Read the model definition and answer for the solid it produces. Units are mm, in the model's axes. Coordinates: 2 decimals unless noted, no trailing zeros. Order: outer loops, then holes, each group sorted by start corner. A loop starts at its lowest first (then second) coordinate and runs counter-clockwise, first axis right, second up.
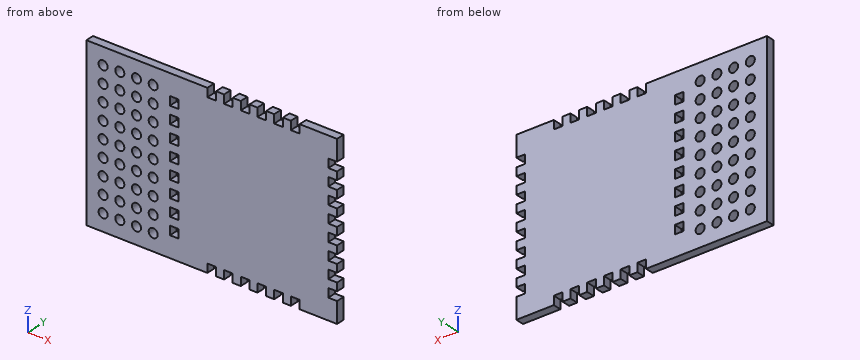
```python
from build123d import *

# Parameters (mm, degrees)
SKETCH1_W           = 127
SKETCH1_H           = 127
BOSS_EXTRUDE1_DEPTH = 6.35
SKETCH2_W           = 6.604
SKETCH2_H           = 6.477
SKETCH2_H_2         = 6.604
CUT_EXTRUDE1_DEPTH  = 91.02678768
SKETCH3_W           = 63.5
SKETCH3_H           = 127
SKETCH3_R           = 3.429
BOSS_EXTRUDE2_DEPTH = 6.35


with BuildPart() as part:
    # Sketch1 → Boss-Extrude1 (new body)
    with BuildSketch(Plane(origin=(0, 0, 0), x_dir=(1, 0, 0), z_dir=(0, 1, 0))):
        Rectangle(SKETCH1_W, SKETCH1_H)
    extrude(amount=BOSS_EXTRUDE1_DEPTH)

    # Sketch2 → Cut-Extrude1 (cut, through all)
    with BuildSketch(Plane(origin=(0, 6.35, 0), x_dir=(1, 0, 0), z_dir=(0, 1, 0))):
        with Locations((-31.75, -60.2615)):
            Rectangle(SKETCH2_W, SKETCH2_H)
        with Locations((-19.05, -60.2615)):
            Rectangle(SKETCH2_W, SKETCH2_H)
        with Locations((-6.35, -60.2615)):
            Rectangle(SKETCH2_W, SKETCH2_H)
        with Locations((6.35, -60.2615)):
            Rectangle(SKETCH2_W, SKETCH2_H)
        with Locations((19.05, -60.2615)):
            Rectangle(SKETCH2_W, SKETCH2_H)
        with Locations((31.75, -60.2615)):
            Rectangle(SKETCH2_W, SKETCH2_H)
        with Locations((31.75, 60.2615)):
            Rectangle(SKETCH2_W, SKETCH2_H)
        with Locations((19.05, 60.2615)):
            Rectangle(SKETCH2_W, SKETCH2_H)
        with Locations((6.35, 60.2615)):
            Rectangle(SKETCH2_W, SKETCH2_H)
        with Locations((-6.35, 60.2615)):
            Rectangle(SKETCH2_W, SKETCH2_H)
        with Locations((-19.05, 60.2615)):
            Rectangle(SKETCH2_W, SKETCH2_H)
        with Locations((-31.75, 60.2615)):
            Rectangle(SKETCH2_W, SKETCH2_H)
        with Locations((-60.198, 31.75)):
            Rectangle(SKETCH2_W, SKETCH2_H_2)
        with Locations((-60.198, 19.05)):
            Rectangle(SKETCH2_W, SKETCH2_H_2)
        with Locations((-60.198, 6.35)):
            Rectangle(SKETCH2_W, SKETCH2_H_2)
        with Locations((-60.198, -6.35)):
            Rectangle(SKETCH2_W, SKETCH2_H_2)
        with Locations((-60.198, -19.05)):
            Rectangle(SKETCH2_W, SKETCH2_H_2)
        with Locations((-60.198, -31.75)):
            Rectangle(SKETCH2_W, SKETCH2_H_2)
        with Locations((60.198, -31.75)):
            Rectangle(SKETCH2_W, SKETCH2_H_2)
        with Locations((60.198, -19.05)):
            Rectangle(SKETCH2_W, SKETCH2_H_2)
        with Locations((60.198, -6.35)):
            Rectangle(SKETCH2_W, SKETCH2_H_2)
        with Locations((60.198, 6.35)):
            Rectangle(SKETCH2_W, SKETCH2_H_2)
        with Locations((60.198, 19.05)):
            Rectangle(SKETCH2_W, SKETCH2_H_2)
        with Locations((60.198, 31.75)):
            Rectangle(SKETCH2_W, SKETCH2_H_2)
        with Locations((-60.198, 44.45)):
            Rectangle(SKETCH2_W, SKETCH2_H_2)
        with Locations((-60.198, -44.45)):
            Rectangle(SKETCH2_W, SKETCH2_H_2)
        with Locations((60.198, -44.45)):
            Rectangle(SKETCH2_W, SKETCH2_H_2)
        with Locations((60.198, 44.45)):
            Rectangle(SKETCH2_W, SKETCH2_H_2)
    extrude(amount=-CUT_EXTRUDE1_DEPTH, mode=Mode.SUBTRACT)

    # Sketch3 → Boss-Extrude2 (add)
    with BuildSketch(Plane(origin=(0, 6.35, 0), x_dir=(1, 0, 0), z_dir=(0, 1, 0))):
        with Locations((-95.25, 0)):
            Rectangle(SKETCH3_W, SKETCH3_H)
        with Locations(Location((-114.3, 50.8, 0), (0, 0, 270))):
            Circle(SKETCH3_R, mode=Mode.SUBTRACT)
        with Locations(Location((-101.6, 50.8, 0), (0, 0, 270))):
            Circle(SKETCH3_R, mode=Mode.SUBTRACT)
        with Locations(Location((-101.6, 38.1, 0), (0, 0, 270))):
            Circle(SKETCH3_R, mode=Mode.SUBTRACT)
        with Locations(Location((-114.3, 38.1, 0), (0, 0, 270))):
            Circle(SKETCH3_R, mode=Mode.SUBTRACT)
        with Locations(Location((-114.3, 25.4, 0), (0, 0, 270))):
            Circle(SKETCH3_R, mode=Mode.SUBTRACT)
        with Locations(Location((-101.6, 25.4, 0), (0, 0, 270))):
            Circle(SKETCH3_R, mode=Mode.SUBTRACT)
        with Locations(Location((-88.9, 50.8, 0), (0, 0, 270))):
            Circle(SKETCH3_R, mode=Mode.SUBTRACT)
        with Locations(Location((-76.2, 50.8, 0), (0, 0, 270))):
            Circle(SKETCH3_R, mode=Mode.SUBTRACT)
        with Locations(Location((-88.9, 38.1, 0), (0, 0, 270))):
            Circle(SKETCH3_R, mode=Mode.SUBTRACT)
        with Locations(Location((-76.2, 38.1, 0), (0, 0, 270))):
            Circle(SKETCH3_R, mode=Mode.SUBTRACT)
        with Locations(Location((-88.9, 25.4, 0), (0, 0, 270))):
            Circle(SKETCH3_R, mode=Mode.SUBTRACT)
        with Locations(Location((-76.2, 25.4, 0), (0, 0, 270))):
            Circle(SKETCH3_R, mode=Mode.SUBTRACT)
        with Locations(Location((-114.3, 12.7, 0), (0, 0, 270))):
            Circle(SKETCH3_R, mode=Mode.SUBTRACT)
        with Locations(Location((-101.6, 12.7, 0), (0, 0, 270))):
            Circle(SKETCH3_R, mode=Mode.SUBTRACT)
        with Locations(Location((-88.9, 12.7, 0), (0, 0, 270))):
            Circle(SKETCH3_R, mode=Mode.SUBTRACT)
        with Locations(Location((-76.2, 12.7, 0), (0, 0, 270))):
            Circle(SKETCH3_R, mode=Mode.SUBTRACT)
        with Locations(Location((-114.3, 0, 0), (0, 0, 270))):
            Circle(SKETCH3_R, mode=Mode.SUBTRACT)
        with Locations(Location((-101.6, 0, 0), (0, 0, 270))):
            Circle(SKETCH3_R, mode=Mode.SUBTRACT)
        with Locations(Location((-88.9, 0, 0), (0, 0, 270))):
            Circle(SKETCH3_R, mode=Mode.SUBTRACT)
        with Locations(Location((-76.2, 0, 0), (0, 0, 270))):
            Circle(SKETCH3_R, mode=Mode.SUBTRACT)
        with Locations(Location((-114.3, -12.7, 0), (0, 0, 270))):
            Circle(SKETCH3_R, mode=Mode.SUBTRACT)
        with Locations(Location((-101.6, -12.7, 0), (0, 0, 270))):
            Circle(SKETCH3_R, mode=Mode.SUBTRACT)
        with Locations(Location((-88.9, -12.7, 0), (0, 0, 270))):
            Circle(SKETCH3_R, mode=Mode.SUBTRACT)
        with Locations(Location((-76.2, -12.7, 0), (0, 0, 270))):
            Circle(SKETCH3_R, mode=Mode.SUBTRACT)
        with Locations(Location((-114.3, -25.4, 0), (0, 0, 270))):
            Circle(SKETCH3_R, mode=Mode.SUBTRACT)
        with Locations(Location((-101.6, -25.4, 0), (0, 0, 270))):
            Circle(SKETCH3_R, mode=Mode.SUBTRACT)
        with Locations(Location((-88.9, -25.4, 0), (0, 0, 270))):
            Circle(SKETCH3_R, mode=Mode.SUBTRACT)
        with Locations(Location((-76.2, -25.4, 0), (0, 0, 270))):
            Circle(SKETCH3_R, mode=Mode.SUBTRACT)
        with Locations(Location((-114.3, -38.1, 0), (0, 0, 270))):
            Circle(SKETCH3_R, mode=Mode.SUBTRACT)
        with Locations(Location((-101.6, -38.1, 0), (0, 0, 270))):
            Circle(SKETCH3_R, mode=Mode.SUBTRACT)
        with Locations(Location((-88.9, -38.1, 0), (0, 0, 270))):
            Circle(SKETCH3_R, mode=Mode.SUBTRACT)
        with Locations(Location((-76.2, -38.1, 0), (0, 0, 270))):
            Circle(SKETCH3_R, mode=Mode.SUBTRACT)
        with Locations(Location((-114.3, -50.8, 0), (0, 0, 270))):
            Circle(SKETCH3_R, mode=Mode.SUBTRACT)
        with Locations(Location((-101.6, -50.8, 0), (0, 0, 270))):
            Circle(SKETCH3_R, mode=Mode.SUBTRACT)
        with Locations(Location((-88.9, -50.8, 0), (0, 0, 270))):
            Circle(SKETCH3_R, mode=Mode.SUBTRACT)
        with Locations(Location((-76.2, -50.8, 0), (0, 0, 270))):
            Circle(SKETCH3_R, mode=Mode.SUBTRACT)
    extrude(amount=-BOSS_EXTRUDE2_DEPTH)


solid = part.part
```
1) Flat-ended cylindrical pins translate along their axes: pin 1 Ø1 at (x, y) = (30.5, 3.5) entering from +Z; pin 2 Ø4 at (x, z) = (-101.6, 38.1) entering from +Y; pin 3 Ø3 at (y, z) = (2.5, 20) entering from +X. Find the tip coordinate at first contact, or state that the pin passes through.
A:
pin 1: stops at z = 57.02
pin 2: passes through
pin 3: stops at x = 56.9
2) A cutting plane is placed at D-D, the plane x = -32. Determine the outline of the cut face in (y, z), and give its area (3 significant figures).
A:
outline: (0, -57.02) - (6.35, -57.02) - (6.35, 57.02) - (0, 57.02) - close
area: 724 mm2
3) A cutting plane is placed at B-B, the plane z = 19. Determine the outline of the cut face in (x, y), and give its area (3 significant figures).
A:
outline: (-127, 0) - (-63.5, 0) - (-63.5, 6.35) - (-127, 6.35) - close; (-56.9, 0) - (56.9, 0) - (56.9, 6.35) - (-56.9, 6.35) - close
area: 1,130 mm2
4) Straight lines are drawn through the part: line 1 (X direction, y = 1.75, z = -25.4); line 2 (X direction, y = 2, z = -44.5); line 3 (X direction, y = 4.75, z = -27). For each, find the intervals that lie inside material, in ascending order.
A:
line 1: x = -127 to -117.73, -110.87 to -105.03, -98.17 to -92.33, -85.47 to -79.63, -72.77 to 63.5
line 2: x = -127 to -63.5, -56.9 to 56.9
line 3: x = -127 to -117.33, -111.27 to -104.63, -98.57 to -91.93, -85.87 to -79.23, -73.17 to 63.5
5) A cutting plane is placed at C-C, the plane y = 3.25. State how many separate pieces and enclosed holes the cut face has, and give its area (3 significant figures).
A:
separate pieces: 1
enclosed holes: 44
area: 21,700 mm2
6) A cutting plane is placed at A-A, the plane z = 38.1. Determine the outline of the cut face in (x, y).
A:
outline: (-127, 0) - (-117.73, 0) - (-117.73, 6.35) - (-127, 6.35) - close; (-110.87, 0) - (-105.03, 0) - (-105.03, 6.35) - (-110.87, 6.35) - close; (-98.17, 0) - (-92.33, 0) - (-92.33, 6.35) - (-98.17, 6.35) - close; (-85.47, 0) - (-79.63, 0) - (-79.63, 6.35) - (-85.47, 6.35) - close; (-72.77, 0) - (63.5, 0) - (63.5, 6.35) - (-72.77, 6.35) - close
